The drawing under review shows one solid part. Ordinate dimensions are in mm from its lowest x, y, z. Coordinates: 2 decimals unless noted, no trailing zeros. Order: outer loops, then holes, each group sorted by start corner. A loop starts at its lowest first (then second) coordinate and runs counter-clockwise, first axis right, second up.
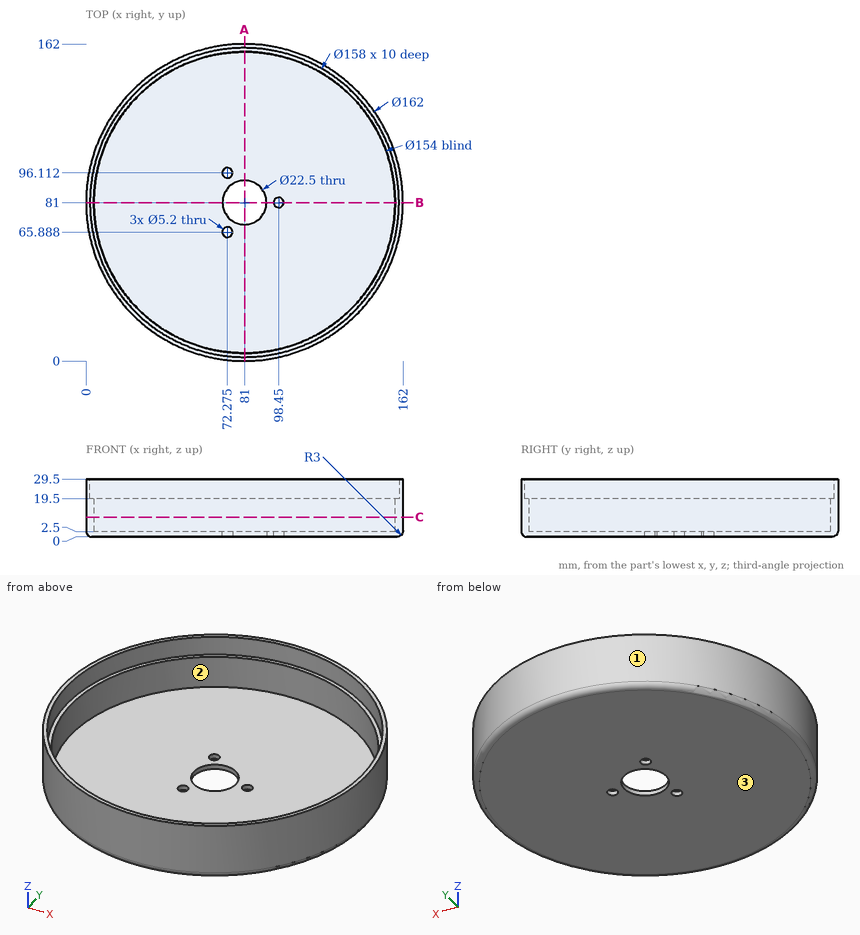
(1) Consider section B-B (y = 81). Give the boundary of the cut face in (x, z), then the cut area to 3 significant figures.
(2) The part is to be moulded in two halves that separate along X. For the marked faces 1, 2 and 3, say which applies: +X half, -X half, draft (parallel to the pull), parting line (faces both ways), or undercut.
(3) Wall thickness on line 1 (Y direction, x = 81, z = 23.5); line 2 (Y direction, x = 128, z = 4.75); line 3 (Z direction, x = 80, y = 45): over which ranges is each line inside the solid? List them lowest first.
(4) Consider section C-C (z = 10). Give the boundary of the cut face in (x, y).
(5) Consider section A-A (x = 81). Give the boundary of the cut face in (y, z), then the cut area to 3 significant figures.
(6) Insertion check: pin 1 Ø1.5 at (x, y) = (51.5, 65.5) entering from +Z; pin 2 Ø5 at (y, z) = (58.5, 16) entering from -X; pin 3 Ø18 at (x, y) = (81, 81) entering from -Z; pin 4 Ø10 at (y, z) = (90, 19.5) entering from -X. Each pin has a flat end and moves straight along its axis. Give the tip position at first contact, or say it passes through.
Findings:
1. outline: (0, 3) arc R3 ccw to (3, 0) - (69.75, 0) - (69.75, 2.5) - (4, 2.5) - (4, 19.5) - (2, 19.5) - (2, 29.5) - (0, 29.5) - close; (92.25, 0) - (95.85, 0) - (95.85, 2.5) - (92.25, 2.5) - close; (101.05, 0) - (159, 0) arc R3 ccw to (162, 3) - (162, 29.5) - (160, 29.5) - (160, 19.5) - (158, 19.5) - (158, 2.5) - (101.05, 2.5) - close
1. area: 508 mm2
2. face 1: parting line
2. face 2: undercut
2. face 3: draft
3. line 1: y = 0 to 2, 160 to 162
3. line 2: y = 15.03 to 20.01, 141.99 to 146.97
3. line 3: z = 0 to 2.5
4. outline: circle Ø162 at (81, 81); hole circle Ø154 at (81, 81)
5. outline: (0, 3) arc R3 ccw to (3, 0) - (69.75, 0) - (69.75, 2.5) - (4, 2.5) - (4, 19.5) - (2, 19.5) - (2, 29.5) - (0, 29.5) - close; (92.25, 0) - (159, 0) arc R3 ccw to (162, 3) - (162, 29.5) - (160, 29.5) - (160, 19.5) - (158, 19.5) - (158, 2.5) - (92.25, 2.5) - close
5. area: 521 mm2
6. pin 1: stops at z = 2.5
6. pin 2: stops at x = 2.51
6. pin 3: passes through
6. pin 4: stops at x = 0.1
